Here's how the part is built. I have some questions about the finished solid (model axes, mm). A direction names the side the tool comes from. Give positions to 0.01 mm unless a question says otherwise; leave off trailing zeros. Order: outer loops, then holes, each group sorted by start corner. A loop starts at its lowest first (then second) coordinate and runs counter-clockwise, first axis right, second up.
from build123d import *

# Parameters (mm, degrees)
SKETCH1_W           = 10
SKETCH1_H           = 4
SKETCH1_W_2         = 4
SKETCH1_H_2         = 10
BOSS_EXTRUDE1_DEPTH = 4


with BuildPart() as part:
    # Sketch1 → Boss-Extrude1 (new body)
    with BuildSketch(Plane(origin=(0, 0, 0), x_dir=(1, 0, 0), z_dir=(0, 1, 0))):
        Polygon((4, 10), (4, 4), (10, 4), (20, 4), (26, 4), (26, 10), (26, 20), (26, 26), (20, 26), (10, 26), (4, 26), (4, 20), align=None)
        with Locations((15, 2)):
            Rectangle(SKETCH1_W, SKETCH1_H)
        with Locations((28, 15)):
            Rectangle(SKETCH1_W_2, SKETCH1_H_2)
        with Locations((15, 28)):
            Rectangle(SKETCH1_W, SKETCH1_H)
        with Locations((2, 15)):
            Rectangle(SKETCH1_W_2, SKETCH1_H_2)
    extrude(amount=BOSS_EXTRUDE1_DEPTH)


solid = part.part
Q1. If we section it at C-C on x = 2.5: List the corners of the cut face in (y, z) for me.
Filled sheet:
outline: (0, -20) - (4, -20) - (4, -10) - (0, -10) - close
Q2. If we section it at A-A on y = 2.1: List the corners of the cut face in (x, z) for me, plus the area to 3 significant figures.
Filled sheet:
outline: (0, -20) - (4, -20) - (4, -26) - (10, -26) - (10, -30) - (20, -30) - (20, -26) - (26, -26) - (26, -20) - (30, -20) - (30, -10) - (26, -10) - (26, -4) - (20, -4) - (20, 0) - (10, 0) - (10, -4) - (4, -4) - (4, -10) - (0, -10) - close
area: 644 mm2
Q3. If we section it at B-B on z = -6.25: List the corners of the cut face in (x, y) for me.
Filled sheet:
outline: (4, 0) - (26, 0) - (26, 4) - (4, 4) - close
Q4. I'm going to push flat-ended pins straight in: P1, Ø2, axis at y = 1, z = -6, coming from the +X side; P2, Ø2, axis at y = 2.5, z = -2, coming from the -X side; P3, Ø1.2, axis at x = 27.5, y = 2, coming from the -Z side. Where does each tip first touch, or does it pass through?
Filled sheet:
P1: stops at x = 26
P2: stops at x = 10
P3: stops at z = -20
Q5. For faces 1 (the face through (20, 2, -28)), 2 (the face through (7, 2, -26)), 3 (the face through (0, 2, -15)), 4 (the face through (23, 2, -4)), 5 (the face through (4, 2, -7)), which set-ups out of +Z, -Z, +X, -X, +Y, -Y let a thin tool reach every point of the face, with its end or its side?
Filled sheet:
face 1: -Z, +X, +Y, -Y
face 2: -Z, -X, +Y, -Y
face 3: +Z, -Z, -X, +Y, -Y
face 4: +Z, +X, +Y, -Y
face 5: +Z, -X, +Y, -Y
Q6. I need wall thicknesses on L1, parallel to X at y = 1.25, z = -20.75; L2, parallel to X at y = 1.2, z = -28.25; L3, parallel to Z at x = 24.5, y = 3.5. Which ranges of each line are inside material? Lowest first, please.
Filled sheet:
L1: x = 4 to 26
L2: x = 10 to 20
L3: z = -26 to -4
